```python
from build123d import *

# Parameters (mm, degrees)
SKETCH1_W                = 30
SKETCH1_H                = 30
BOSS_EXTRUDE1_DEPTH      = 8
SKETCH5_R                = 1.45
CUT_EXTRUDE3_DEPTH       = 23.671568098
LPATTERN1_COUNT          = 6
LPATTERN1_PITCH          = 5
LPATTERN1_COUNT_DIR2     = 6
LPATTERN1_PITCH_DIR2     = 5
BOSS_EXTRUDE2_DEPTH      = 2
BOSS_EXTRUDE2_DEPTH_BACK = 8
SKETCH2_R                = 2.5
SKETCH3_R                = 0.975
CUT_EXTRUDE1_DEPTH       = 24.452078799
SKETCH4_W                = 12
SKETCH4_H                = 4
CUT_EXTRUDE2_DEPTH       = 23.671568098
CHAMFER1_SIZE            = 2


with BuildPart() as part:
    # Sketch1 → Boss-Extrude1 (new body)
    with BuildSketch(Plane(origin=(0, 0, 0), x_dir=(1, 0, 0), z_dir=(0, 1, 0))):
        Rectangle(SKETCH1_W, SKETCH1_H)
    extrude(amount=BOSS_EXTRUDE1_DEPTH)

    # Sketch5 → Cut-Extrude3 (cut, through all)
    with BuildSketch(Plane.XZ):
        with Locations(Location((-12.5, 12.5, 0), (0, 0, 270))):
            Circle(SKETCH5_R)
    cut_extrude3 = extrude(amount=-CUT_EXTRUDE3_DEPTH, mode=Mode.SUBTRACT)

    # LPattern1: Cut-Extrude3 6 × 6, 10 skipped
    with Locations(*[(i * LPATTERN1_PITCH, 0, -j * LPATTERN1_PITCH_DIR2) for i in range(LPATTERN1_COUNT) for j in range(LPATTERN1_COUNT_DIR2) if (i, j) not in ((0, 0), (0, 1), (0, 4), (1, 0), (1, 5), (2, 5), (3, 5), (4, 0), (4, 5), (5, 1), (5, 4))]):
        add(cut_extrude3, mode=Mode.SUBTRACT)

    # Sketch2 → Boss-Extrude2 (add, two sides: drawn at the far end of the back side and taken through both)
    with BuildSketch(Plane(origin=(0, 8, 0), x_dir=(1, 0, 0), z_dir=(0, 1, 0)).offset(-BOSS_EXTRUDE2_DEPTH_BACK)):
        with Locations(Location((-11.65, 11.9, 0), (0, 0, 270))):
            Circle(SKETCH2_R)
        with Locations(Location((11.65, 11.9, 0), (0, 0, 270))):
            Circle(SKETCH2_R)
        with Locations(Location((11.65, -11.9, 0), (0, 0, 270))):
            Circle(SKETCH2_R)
        with Locations(Location((-11.65, -11.9, 0), (0, 0, 270))):
            Circle(SKETCH2_R)
    extrude(amount=BOSS_EXTRUDE2_DEPTH + BOSS_EXTRUDE2_DEPTH_BACK)

    # Sketch3 → Cut-Extrude1 (cut, through all)
    with BuildSketch(Plane(origin=(0, 10, 0), x_dir=(1, 0, 0), z_dir=(0, 1, 0))):
        with Locations(Location((-11.65, 11.9, 0), (0, 0, 270))):
            Circle(SKETCH3_R)
        with Locations(Location((11.65, 11.9, 0), (0, 0, 270))):
            Circle(SKETCH3_R)
        with Locations(Location((-11.65, -11.9, 0), (0, 0, 270))):
            Circle(SKETCH3_R)
        with Locations(Location((11.65, -11.9, 0), (0, 0, 270))):
            Circle(SKETCH3_R)
    extrude(amount=-CUT_EXTRUDE1_DEPTH, mode=Mode.SUBTRACT)

    # Sketch4 → Cut-Extrude2 (cut, through all)
    with BuildSketch(Plane(origin=(0, 8, 0), x_dir=(1, 0, 0), z_dir=(0, 1, 0))):
        with Locations((0, 13)):
            Rectangle(SKETCH4_W, SKETCH4_H)
    extrude(amount=-CUT_EXTRUDE2_DEPTH, mode=Mode.SUBTRACT)

    # Chamfer1
    # the kernel refuses this chamfer: 2 mm, written as the material it adds along each edge
    with BuildSketch(Plane(origin=(-11.65, 8, -11.9), x_dir=(0, 0, 1), z_dir=(-1, 0, 0))) as chamfer1_piece_1_section:
        Polygon((2.5 + CHAMFER1_SIZE, 0), (2.5, CHAMFER1_SIZE), (2.5, 0), align=None)
    chamfer1_piece_1 = revolve(axis=Axis((-11.65, 8, -11.9), (0, 1, 0)), mode=Mode.PRIVATE)
    chamfer1_piece_1 = split(chamfer1_piece_1, bisect_by=Plane(origin=(-8.021209726, 8.262551845, -15), z_dir=(0, 0, 1)), keep=Keep.TOP, mode=Mode.PRIVATE)
    chamfer1_piece_1 = split(chamfer1_piece_1, bisect_by=Plane(origin=(-15, 8.262551845, -9.804916959), z_dir=(1, 0, 0)), keep=Keep.TOP, mode=Mode.PRIVATE)
    chamfer1_piece_1 = split(chamfer1_piece_1, bisect_by=Plane(origin=(-8.021209726, 10, -9.804916959), z_dir=(0, -1, 0)), keep=Keep.TOP, mode=Mode.PRIVATE)
    add(chamfer1_piece_1)
    with BuildSketch(Plane(origin=(11.65, 8, -11.9), x_dir=(0, 0, 1), z_dir=(-1, 0, 0))) as chamfer1_piece_2_section:
        Polygon((2.5 + CHAMFER1_SIZE, 0), (2.5, CHAMFER1_SIZE), (2.5, 0), align=None)
    chamfer1_piece_2 = revolve(axis=Axis((11.65, 8, -11.9), (0, 1, 0)), mode=Mode.PRIVATE)
    chamfer1_piece_2 = split(chamfer1_piece_2, bisect_by=Plane(origin=(15, 8.948074694, -10.147678382), z_dir=(-1, 0, 0)), keep=Keep.TOP, mode=Mode.PRIVATE)
    chamfer1_piece_2 = split(chamfer1_piece_2, bisect_by=Plane(origin=(14.685110074, 8.948074694, -15), z_dir=(0, 0, 1)), keep=Keep.TOP, mode=Mode.PRIVATE)
    chamfer1_piece_2 = split(chamfer1_piece_2, bisect_by=Plane(origin=(14.685110074, 10, -10.147678382), z_dir=(0, -1, 0)), keep=Keep.TOP, mode=Mode.PRIVATE)
    add(chamfer1_piece_2)
    with BuildSketch(Plane(origin=(11.65, 8, 11.9), x_dir=(0, 0, 1), z_dir=(-1, 0, 0))) as chamfer1_piece_3_section:
        Polygon((2.5 + CHAMFER1_SIZE, 0), (2.5, CHAMFER1_SIZE), (2.5, 0), align=None)
    chamfer1_piece_3 = revolve(axis=Axis((11.65, 8, 11.9), (0, 1, 0)), mode=Mode.PRIVATE)
    chamfer1_piece_3 = split(chamfer1_piece_3, bisect_by=Plane(origin=(11.65, 8.948074692, 15), z_dir=(0, 0, -1)), keep=Keep.TOP, mode=Mode.PRIVATE)
    chamfer1_piece_3 = split(chamfer1_piece_3, bisect_by=Plane(origin=(15, 8.948074692, 8.395356766), z_dir=(-1, 0, 0)), keep=Keep.TOP, mode=Mode.PRIVATE)
    chamfer1_piece_3 = split(chamfer1_piece_3, bisect_by=Plane(origin=(11.65, 10, 8.395356766), z_dir=(0, -1, 0)), keep=Keep.TOP, mode=Mode.PRIVATE)
    add(chamfer1_piece_3)
    with BuildSketch(Plane(origin=(-11.65, 8, 11.9), x_dir=(0, 0, 1), z_dir=(-1, 0, 0))) as chamfer1_piece_4_section:
        Polygon((2.5 + CHAMFER1_SIZE, 0), (2.5, CHAMFER1_SIZE), (2.5, 0), align=None)
    chamfer1_piece_4 = revolve(axis=Axis((-11.65, 8, 11.9), (0, 1, 0)), mode=Mode.PRIVATE)
    chamfer1_piece_4 = split(chamfer1_piece_4, bisect_by=Plane(origin=(-15, 8.948074692, 8.395356766), z_dir=(1, 0, 0)), keep=Keep.TOP, mode=Mode.PRIVATE)
    chamfer1_piece_4 = split(chamfer1_piece_4, bisect_by=Plane(origin=(-11.65, 8.948074692, 15), z_dir=(0, 0, -1)), keep=Keep.TOP, mode=Mode.PRIVATE)
    chamfer1_piece_4 = split(chamfer1_piece_4, bisect_by=Plane(origin=(-11.65, 10, 8.395356766), z_dir=(0, -1, 0)), keep=Keep.TOP, mode=Mode.PRIVATE)
    add(chamfer1_piece_4)


solid = part.part
```
Here's how the part is built. I have some questions about the finished solid (model axes, mm). A direction names the side the tool comes from. Give positions to 0.01 mm unless a question says otherwise; leave off trailing zeros. Write each loop counter-clockwise with the first axis right and the second up, starting at its lowest first coordinate (ties: lowest second). Pieces come first, ordered by that corner, then holes. Notation, with made-up numbers: M 1,26.25 L 20,26.25 A19 cw 20,63.25 Z; hole C -18.75,33 d4. An arc over 180 degrees is marked long. Put each result on its own line as item: value. Start each with the question number.
Item 1: If we section it at C-C, the plane y = 4.25: Count the separate pieces of the cut face and the enclosed holes in it, then the cut area to 3 significant figures.
Item 2: Will these pins go through, and if not, where does the flat tip stop? pin 1 (4 mm diameter, centred on x = -7.5, z = 7.5, fed in from +Y); pin 2 (1.7 mm diameter, centred on x = -2.5, z = -2.5, fed in from +Y); pin 3 (3.5 mm diameter, centred on x = -2.5, z = 12.5, fed in from +Y); pin 4 (6 mm diameter, centred on x = -2, y = 2.5, fed in from -Z).
Item 3: If we section it at A-A, the plane z = -2.5: Write out the boundary of the cut face in (x, y).
Item 4: Thinking about a two-plate mould opening in X: for faces 1 (the flat face through (0, 8, 0)), 2 (the flat face through (12, 10, 13)), which applies, +X half, -X half, draft (parallel to the pull), parting line (faces both ways), or undercut?
Item 5: If we section it at D-D, the plane z = -11.9: Write out the boundary of the cut face in (x, y) (3 decimals), then the cut area to 3 significant figures.
Item 6: On a 3-axis mill with a long thin cutter (end or side, diameter ignored), from which of +Z, -Z, +X, -X, +Y, -Y can I reach the whole of each face in a straight line? I mean faces 3 (the flat face through (6, 4, -13)), 4 (the cylindrical face through (2.56, 3.94, 8.95)). Say none if no direction works.
Item 7: If we section it at B-B, the plane x = 2.5: Write out the boundary of the cut face in (y, z), then the cut area to 3 significant figures.
Item 8: I need wall thicknesses on L1, parallel to Z at x = -13, y = 2; L2, parallel to Z at x = -3.25, y = 7; L3, parallel to Z at x = 6.5, y = 6.25. Which ranges of each line are inside material? Lowest first, please. Write a range as from..to.
Values:
1. separate pieces: 1
1. enclosed holes: 26
1. area: 695 mm²
2. pin 1: y = 8.45
2. pin 2: through
2. pin 3: y = 8
2. pin 4: z = -11
3. outline: M -15,0 L -13.95,0 L -13.95,8 L -15,8 Z; M -11.05,0 L -8.95,0 L -8.95,8 L -11.05,8 Z; M -6.05,0 L -3.95,0 L -3.95,8 L -6.05,8 Z; M -1.05,0 L 1.05,0 L 1.05,8 L -1.05,8 Z; M 3.95,0 L 6.05,0 L 6.05,8 L 3.95,8 Z; M 8.95,0 L 11.05,0 L 11.05,8 L 8.95,8 Z; M 13.95,0 L 15,0 L 15,8 L 13.95,8 Z
4. face 1: undercut
4. face 2: draft
5. outline: M -15,0 L -12.625,0 L -12.625,10 L -14.15,10 L -15,9.15 Z; M -10.675,0 L -6,0 L -6,8 L -7.15,8 L -9.15,10 L -10.675,10 Z; M 6,0 L 10.675,0 L 10.675,10 L 9.15,10 L 7.15,8 L 6,8 Z; M 12.625,0 L 15,0 L 15,9.15 L 14.15,10 L 12.625,10 Z
5. area: 132 mm²
6. face 3: -Z, +Y, -Y
6. face 4: +Y, -Y
7. outline: M 0,-11 L 8,-11 L 8,-8.95 L 0,-8.95 Z; M 0,-6.05 L 8,-6.05 L 8,-3.95 L 0,-3.95 Z; M 0,-1.05 L 8,-1.05 L 8,1.05 L 0,1.05 Z; M 0,3.95 L 8,3.95 L 8,6.05 L 0,6.05 Z; M 0,8.95 L 8,8.95 L 8,11.05 L 0,11.05 Z; M 0,13.95 L 8,13.95 L 8,15 L 0,15 Z
7. area: 92.0 mm²
8. L1: -15..-3.86, -1.14..1.14, 3.86..15
8. L2: -11..-8.74, -6.26..-3.74, -1.26..1.26, 3.74..6.26, 8.74..11.26, 13.74..15
8. L3: -15..-8.55, -6.45..-3.55, -1.45..1.45, 3.55..6.45, 8.55..15
